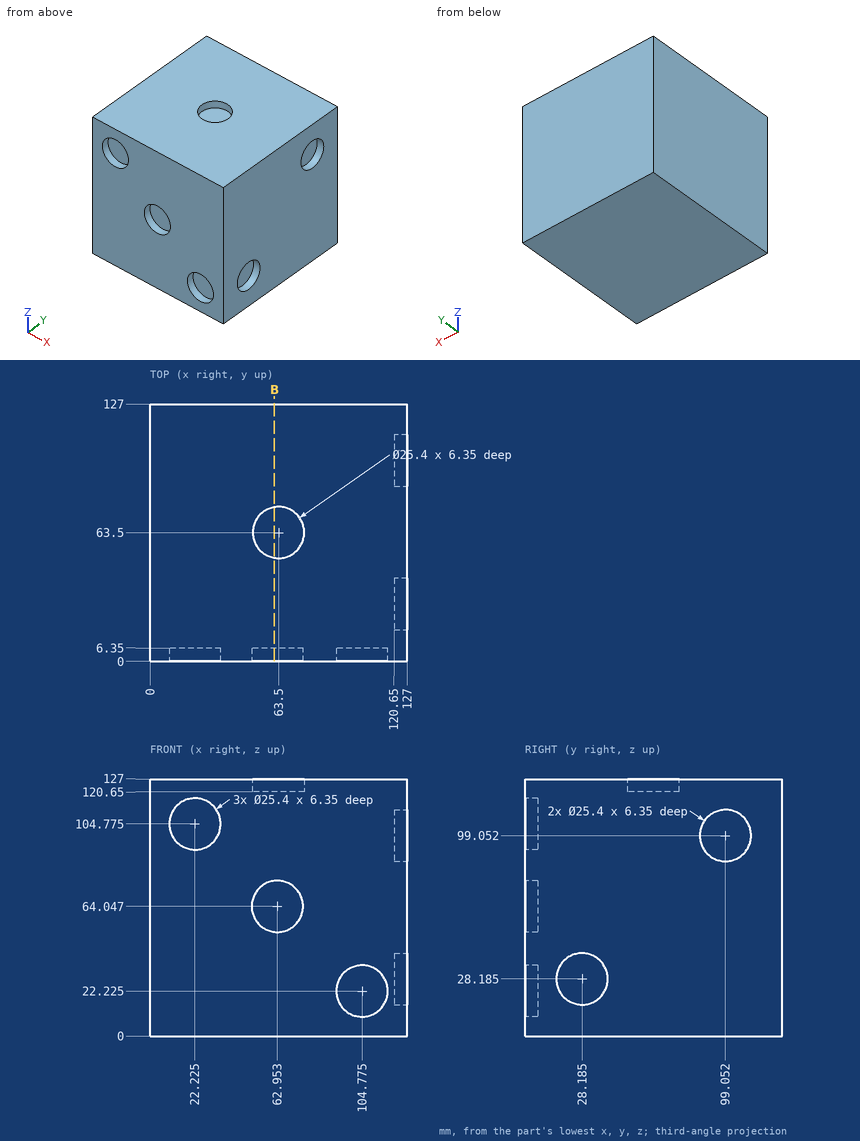
Geometry check sheet. Reference: drawing and pictorial views, mm from the part's lowest x, y, z. Give positions to 0.01 mm unless a question says otherwise; leave off trailing zeros. Order: outer loops, then holes, each group sorted by start corner. A loop starts at its lowest first (then second) coordinate and runs counter-clockwise, first axis right, second up. Notation, with made-up numbers: M 28,66 L 42,66 A9 ccw 42,72 Z; hole C 66.25,33.5 d11. An arc over 180 degrees is marked long. Answer as CSV lines item,"result". Start each with the question number.
Item 1: Cross-section at B-B on x = 61.5. Enter the section's corners in (y, z), plus the area to 3 significant figures.
Item 2: Gauge pin test, flat ends, axial feed: P1, Ø12.5, axis at x = 102.5, z = 19, coming from the -Y side; P2, Ø15, axis at y = 28.19, z = 28.19, coming from the +X side; P3, Ø7.5, axis at x = 67, y = 58.5, coming from the +Z side. Record the tip position at first contact, or that the pin passes through.
Item 3: Thickness scan on line 1 (Y direction, x = 32, z = 107.5); line 2 (X direction, y = 16, z = 31). Record the ranges inside material, lowest first. Write a range as [from, to].
Established:
1,outline,"M 0,0 L 127,0 L 127,127 L 76.04,127 L 76.04,120.65 L 50.96,120.65 L 50.96,127 L 0,127 L 0,76.66 L 6.35,76.66 L 6.35,51.43 L 0,51.43 Z"
1,area,"15,800 mm^2"
2,P1,"stops at y = 6.35"
2,P2,"stops at x = 120.65"
2,P3,"stops at z = 120.65"
3,line 1,"y = [6.35, 127]"
3,line 2,"x = [0, 120.65]"
